Autodesk Inventor part; units mm, degrees
ref_plane "YZ Plane" through (0, 0, 0) normal (1, 0, 0) x (0, 1, 0)
ref_plane "XZ Plane" through (0, 0, 0) normal (0, 1, 0) x (-1, 0, 0)
ref_plane "XY Plane" through (0, 0, 0) normal (0, 0, 1) x (1, 0, 0)
sketch "Sketch1" plane through (0, 0, 0) normal (0, 0, 1) x (1, 0, 0)
  circle A0 centre (0, 0) radius 10
  dimension "Diameter" = 20
extrude "Base" add sketch "Sketch1" along normal mid plane 16
sketch "Sketch3" plane through (0, 0, 0) normal (0, 1, 0) x (-1, 0, 0)
  line L0 (-10, -8) -> (-10, 8)
  line L1 (10, -8) -> (10, 8)
  line L2 (-10, 8) -> (10, 8)
  line L3 (10, -8) -> (-10, -8)
  line L4 (-10, 2.2) -> (0.5164, -8)
  line L5 (-0.5164, -8) -> (10, 2.2)
  line L6 (0, -11.2) -> (0, 11.2) construction
  dimension "d43" = 91.75
  dimension "d44" = 5.8
extrude "Pneumatic Cut" [suppressed]
sketch "Sketch2" plane through (0, 0, 8) normal (0, 0, 1) x (1, 0, 0)
  circle A0 centre (0, 0) radius 10
  line L0 (-4, 9.1652) -> (4, 9.1652)
  line L1 (4, 9.1652) -> (4, 23.8)
  line L2 (4, 23.8) -> (-4, 23.8)
  line L3 (-4, 23.8) -> (-4, 9.1652)
  point P0 (0, 23.8)
  dimension "Tab_Length" = 33.8
  dimension "Tab_Width" = 8
extrude "Tab" add sketch "Sketch2" against normal blind 1 contours A0 L3 L2 L1
hole "M6 Thru Hole" [suppressed]
hole "M8 Thru Hole" at (0, -10, 0) direction (0, 1, 0) diameter 9 end through all counterbore diameter 15 counterbore depth 10
hole "M6 Threaded" [suppressed]
hole "M8 Threaded" [suppressed]
equation "\"d21\" = 0.5 * Diameter"
equation "\"d8\" = 0.5 * Diameter"
properties part number "20-004Z1" material "Zinc ZA-12"
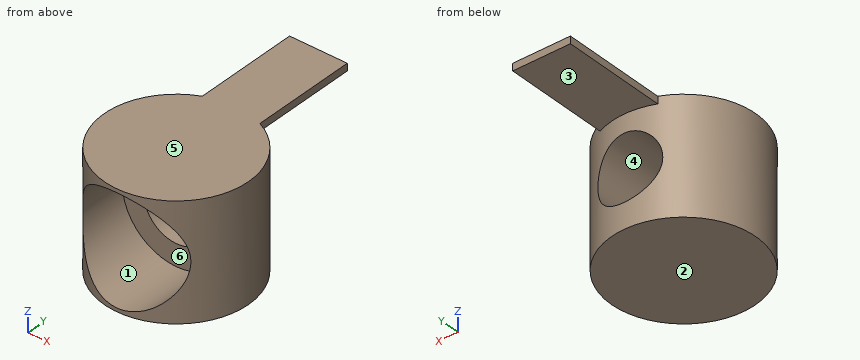
Could you check a few things on this model? Use its own coordinates, in mm. Face numbers are marked on the shaded views. A direction names the side the tool comes from. Coordinates: 2 decimals unless noted, no trailing zeros. Write each loop counter-clockwise with the first axis right and the second up, starting at its lowest first coordinate (ties: lowest second). Pieces come first, ordered by that corner, then holes. Notation, with made-up numbers: (22, -13.75) - (67, -13.75) arc R37 ccw to (67, 22.25) - close; hole circle Ø9 at (30, 45.25). An arc over 180 degrees is marked (long way). Put each result on its own line as item: value. Start each with the question number.
Q1. I'm going to push flat-ended pins straight in: P1, Ø1.1, axis at y = 20, z = 7.5, coming from the +X side; P2, Ø5, axis at x = 6, z = -1.5, coming from the +Y side; P3, Ø9, axis at x = 0.5, y = 19, coming from the -Z side; P4, Ø4, axis at y = -2, z = 2, coming from the +X side. Where does each tip first touch, or does it pass through?
Q2. Which directions (+Z, -Z, +X, -X, +Y, -Y) give clear straight access to the entire face, cutting with the end or side of a thin tool? Please do the marked faces 1 and 2.
Q3. Please list where these lines run through material, in increasing order: L1, parallel to Z at x = 0, y = 5.75; L2, parallel to Z at x = 0, y = -5.5; L3, parallel to X at y = 5.5, z = 0.
Q4. I want a section at D-D on y = 4.5. Write out the boundary of the cut face in (x, z), plus the area to 3 significant figures.
Q5. Thinking about a two-plate mould opening in Z: for the marked faces 3, 4, 5 and 6, which applies, pulls with the +Z half, pulls with the -Z half, needs draft (parallel to the pull), parting line crosses it, or undercut?
Q6. I want a section at C-C on x = 0. Write out the boundary of the cut face in (y, z).
Q7. I want a section at A-A on y = -8. Write out the boundary of the cut face in (x, z), plus the area to 3 significant figures.
Q8. I want a section at B-B on z = 2.5. Write out the boundary of the cut face in (x, y), plus the area to 3 significant figures.
Checks:
1. P1: x = 4
1. P2: y = 9.28
1. P3: z = 7
1. P4: x = 10
2. face 1: -Y
2. face 2: -Z, +X, -X, +Y, -Y
3. L1: -8 to -4.5, 4.5 to 8
3. L2: -8 to -7.5, 7.5 to 8
3. L3: -8.35 to -4.5, 4.5 to 8.35
4. outline: (-8.93, -8) - (8.93, -8) - (8.93, 8) - (-8.93, 8) - close; hole circle Ø9 at (0, 0)
4. area: 222 mm²
5. face 3: pulls with the -Z half
5. face 4: undercut
5. face 5: pulls with the +Z half
5. face 6: undercut
6. outline: (-10, -8) - (10, -8) - (10, -4.5) - (0, -4.5) - (0, -7.5) - (-10, -7.5) - close; (-10, 7.5) - (0, 7.5) - (0, 4.5) - (10, 4.5) - (10, 7) - (23.8, 7) - (23.8, 8) - (-10, 8) - close
7. outline: (-6, -8) - (6, -8) - (6, -4.5) arc R7.5 cw to (-6, -4.5) - close; (-6, 4.5) arc R7.5 cw to (6, 4.5) - (6, 8) - (-6, 8) - close
7. area: 33.7 mm²
8. outline: (-7.07, -7.07) - (-7.07, 0) - (-3.74, 0) - (-3.74, 9.27) arc R10 ccw to start; (3.74, 0) - (7.07, 0) - (7.07, -7.07) arc R10 ccw to (3.74, 9.27) - close
8. area: 113 mm²
